The listing builds one solid part. Answer for the finished solid, in the listing's coordinates (mm). A direction names the side the tool comes from. Round coordinates to 2 decimals unless told otherwise and drop trailing zeros. Write each loop counter-clockwise with the first axis right and the second up, starting at its lowest first coordinate (ties: lowest second). Pieces come first, ordered by that corner, then holes. Notation, with made-up numbers: M 81,-5.5 L 113,-5.5 A15 cw 113,23.5 Z; hole C 59.5,9 d3. An arc over 180 degrees is marked long. Answer as CSV lines item,"result". Start each with the question number.
from build123d import *

# Parameters (mm, degrees)
SKETCH1_W           = 190.5
SKETCH1_H           = 50.8
BOSS_EXTRUDE1_DEPTH = 6.35
SKETCH2_W           = 6.35
SKETCH2_H           = 12.7
CUT_EXTRUDE1_DEPTH  = 7.35
SKETCH3_W           = 6.35
SKETCH3_H           = 6.35
CUT_EXTRUDE2_DEPTH  = 7.35
SKETCH4_W           = 12.7
SKETCH4_H           = 6.35
CUT_EXTRUDE3_DEPTH  = 7.35
LPATTERN1_COUNT     = 7
LPATTERN1_PITCH     = 25.4
SKETCH5_W           = 15.875
SKETCH5_H           = 15.875
CUT_EXTRUDE4_DEPTH  = 7.35


with BuildPart() as part:
    # Sketch1 → Boss-Extrude1 (new body)
    with BuildSketch(Plane.XY):
        Rectangle(SKETCH1_W, SKETCH1_H)
    extrude(amount=BOSS_EXTRUDE1_DEPTH)

    # Sketch2 → Cut-Extrude1 (cut, through all)
    with BuildSketch(Plane.XY.offset(6.35)):
        with Locations((-92.075, 0)):
            Rectangle(SKETCH2_W, SKETCH2_H)
    cut_extrude1 = extrude(amount=-CUT_EXTRUDE1_DEPTH, mode=Mode.SUBTRACT)

    # Sketch3 → Cut-Extrude2 (cut, through all)
    with BuildSketch(Plane.XY.offset(6.35)):
        with Locations((-92.075, -22.225)):
            Rectangle(SKETCH3_W, SKETCH3_H)
    cut_extrude2 = extrude(amount=-CUT_EXTRUDE2_DEPTH, mode=Mode.SUBTRACT)

    # Mirror1: Cut-Extrude2 across plane
    add(cut_extrude2.mirror(Plane(origin=(0, 0, 0), x_dir=(0, 0, 1), z_dir=(1, 0, 0))), mode=Mode.SUBTRACT)

    # Mirror2: Cut-Extrude1 across plane
    add(cut_extrude1.mirror(Plane(origin=(0, 0, 0), x_dir=(0, 0, 1), z_dir=(1, 0, 0))), mode=Mode.SUBTRACT)

    # Sketch4 → Cut-Extrude3 (cut, through all)
    with BuildSketch(Plane.XY.offset(6.35)):
        with Locations((-76.2, 22.225)):
            Rectangle(SKETCH4_W, SKETCH4_H)
    cut_extrude3 = extrude(amount=-CUT_EXTRUDE3_DEPTH, mode=Mode.SUBTRACT)

    # LPattern1: Cut-Extrude3 ×7
    with Locations(*[(i * LPATTERN1_PITCH, 0, 0) for i in range(1, LPATTERN1_COUNT)]):
        add(cut_extrude3, mode=Mode.SUBTRACT)

    # Sketch5 → Cut-Extrude4 (cut, through all)
    with BuildSketch(Plane.XY.offset(6.35)):
        with Locations((42.9895, -7.9375)):
            Rectangle(SKETCH5_W, SKETCH5_H)
    extrude(amount=-CUT_EXTRUDE4_DEPTH, mode=Mode.SUBTRACT)


solid = part.part
Q1. Find section A-A (x = -22). Determine the outline of the cut face in (y, z), plus the area to 3 significant figures.
Q2. For faces 1 (the face through (35.052, -8, 3)), 2 (the face through (-44.45, 22, 3)), 3 (the face through (-92, -19.05, 3)), determine the directions among +Z, -Z, +X, -X, +Y, -Y from which every point of the face is accessible in a straight line to the end or side of a thin tool.
Q3. Straight lines are drawn through the part: L1, parallel to X at y = -11.5, z = 0.75; L2, parallel to X at y = -6, z = 5; L3, parallel to Y at x = 38, z = 2.5 (3 decimals). For each, find the intervals that lie inside material, in ascending order.
Q4. Each of these flat-tipped pins is pushed along its axis until it touches: P1, Ø3, axis at x = -22.5, z = 3.5, coming from the +Y side; P2, Ø2, axis at x = 62.5, y = 18.5, coming from the -Z side; P3, Ø3, axis at y = -3, z = 2, coming from the +X side; P4, Ø1, axis at y = -3, z = 3, coming from the -X side. Where does it stop, or does it pass through?
Q5. Find section B-B (y = -21). Determine the outline of the cut face in (x, z).
Reported:
1,outline,"M -25.4,0 L 19.05,0 L 19.05,6.35 L -25.4,6.35 Z"
1,area,"282 mm2"
2,face 1,"+Z, -Z"
2,face 2,"+Z, -Z, +Y"
2,face 3,"+Z, -Z, -X, -Y"
3,L1,"x = -95.25 to 35.05, 50.93 to 95.25"
3,L2,"x = -88.9 to 35.05, 50.93 to 88.9"
3,L3,"y = -25.4 to -15.875, 0 to 25.4"
4,P1,"stops at y = 19.05"
4,P2,"stops at z = 0"
4,P3,"stops at x = 88.9"
4,P4,"stops at x = -88.9"
5,outline,"M -88.9,0 L 88.9,0 L 88.9,6.35 L -88.9,6.35 Z"
